Could you check a few things on this model? Use its own coordinates, in mm. Round coordinates to 2 decimals unless told otherwise and drop trailing zeros. Loops run counter-clockwise (first coordinate to the right, second up) from the corner with the lowest first, then second, coordinate; pieces in that order, holes last. Notation, with made-up numbers: M 17.5,-25 L 59.5,-25 A18 ccw 59.5,-5 Z; hole C -38.5,24.5 d1. An arc over 180 degrees is marked long. Answer in a Markdown table with one row per item.
Autodesk Inventor part; units mm, degrees
ref_plane "Work Plane1" through (65, 0, 0) normal (1, 0, 0) x (0, 1, 0)
ref_plane "Work Plane2" through (0, 87.5, 0) normal (0, 1, 0) x (-1, 0, 0)
ref_plane "XY Plane" through (0, 0, 0) normal (0, 0, 1) x (1, 0, 0)
sketch "Sketch2" plane through (0, 0, 0) normal (0, 0, 1) x (1, 0, 0)
  line L0 (0, 175) -> (130, 175)
  line L1 (130, 175) -> (130, 0)
  line L2 (130, 0) -> (0, 0)
  line L3 (0, 0) -> (0, 175)
  dimension "d2" = 175
  dimension "d3" = 130
extrude "Extrusion1" add sketch "Sketch2" along normal blind 5
sketch "Sketch3" plane through (0, 0, 5) normal (0, 0, 1) x (1, 0, 0)
  line L0 (130, 175) -> (0, 175)
  line L1 (0, 0) -> (130, 0)
  line L2 (0, 175) -> (0, 0)
  line L3 (130, 0) -> (130, 175)
  point P0 (5, 170)
  dimension "d8" = 5
  dimension "d9" = 5
hole "Hole1" at (5, 170, 5) direction (0, 0, -1) diameter 5 depth 5
ref_plane "Work Plane1" through (65, 0, 0) normal (1, 0, 0) x (0, 1, 0)
mirror "Mirror1" about plane through (65, 0, 0) normal (1, 0, 0) of "Hole1"
ref_plane "Work Plane2" through (0, 87.5, 0) normal (0, 1, 0) x (-1, 0, 0)
mirror "Mirror2" about plane through (0, 87.5, 0) normal (0, 1, 0) of "Hole1", "Mirror1"
properties part number "basePlate"
1) I need wall thicknesses on line 1 (X direction, y = 170, z = 1.9). Which ranges of the line are inside material? Lowest first, please.
Computed:
| item | result |
|---|---|
| line 1 | x = 0 to 2.5, 7.5 to 122.5, 127.5 to 130 |
2) I want a section at B-B, the plane y = 170. Please give me the cut outline in (x, z), plus the area to 3 significant figures.
Computed:
| item | result |
|---|---|
| outline | M 0,0 L 2.5,0 L 2.5,5 L 0,5 Z; M 7.5,0 L 122.5,0 L 122.5,5 L 7.5,5 Z; M 127.5,0 L 130,0 L 130,5 L 127.5,5 Z |
| area | 600 mm² |
3) If we mould it in two halves opening along Y, with no side actions, what happens to faces 1 (the face through (127.48, 4.67, 2.46)), 2 (the face through (4.249, 167.615, 2.465)), 3 (the face through (66, 0, 2)), 4 (the face through (0, 86, 2))? For each: released by +Y, released by -Y, zero draft, split by the parting line, or undercut.
Computed:
| item | result |
|---|---|
| face 1 | undercut |
| face 2 | undercut |
| face 3 | released by -Y |
| face 4 | zero draft |
4) I want a section at A-A, the plane x = 5. Please give me the cut outline in (y, z), plus the area to 3 significant figures.
Computed:
| item | result |
|---|---|
| outline | M 0,0 L 2.5,0 L 2.5,5 L 0,5 Z; M 7.5,0 L 167.5,0 L 167.5,5 L 7.5,5 Z; M 172.5,0 L 175,0 L 175,5 L 172.5,5 Z |
| area | 825 mm² |
5) Will this pin go through, and if not, where does the flat tip stop? P1, Ø4, axis at x = 125, y = 5, coming from the +Z side.
Computed:
| item | result |
|---|---|
| P1 | passes through |
